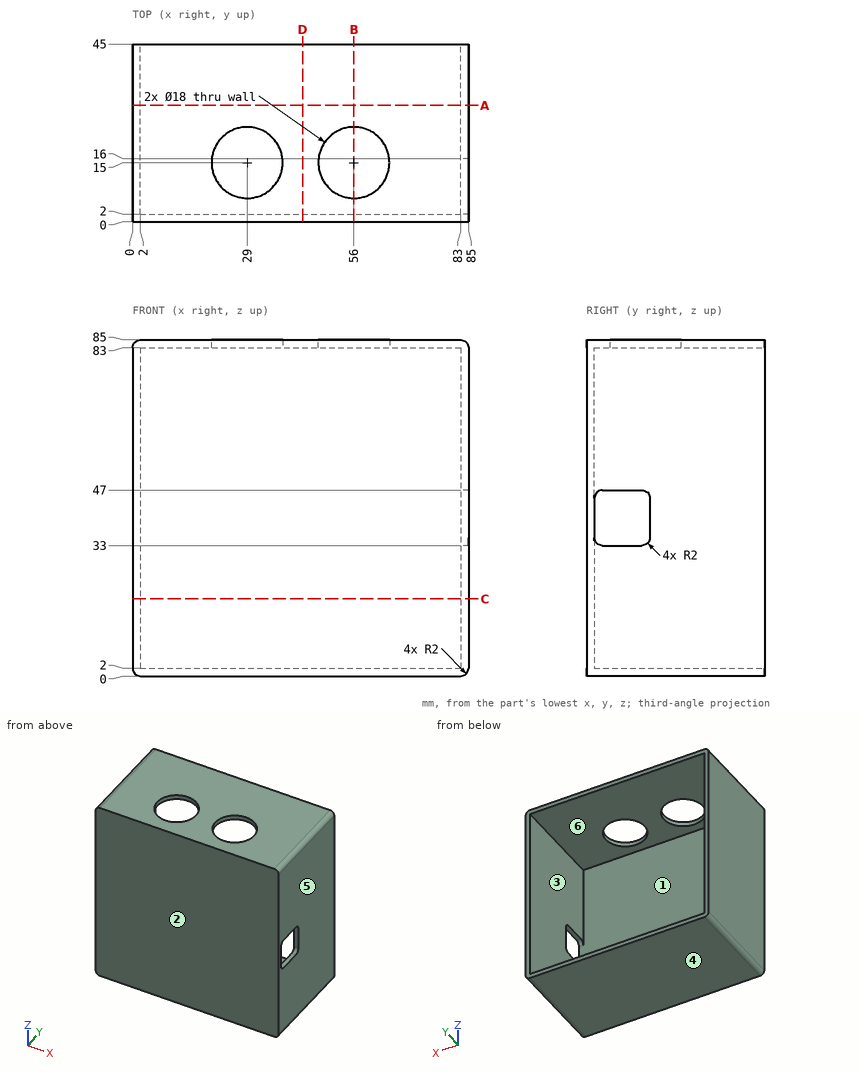
Answer from the drawing. Dimensions are ordinates in mm from the lowest x, y and z of the part. A direction names the side the tool comes from. Give positions to 0.01 mm unless a question says otherwise; leave off trailing zeros. Loops run counter-clockwise (first coordinate to the right, second up) from the corner with the lowest first, then second, coordinate; pieces in that order, holes last. Notation, with made-up numbers: (-19, 39) -> (-11, 39) arc R23 ccw to (-11, 48) -> close; hole circle Ø7 at (72.25, -27). An arc over 180 degrees is marked (long way). One line per question, with ' | ' between items. Start each with the question number.
1) Section C-C, the plane z = 19.5 is taken. Determine the outline of the cut face in (x, y), then the cut area to 3 significant figures.
2) For the marked faces 5 and 6, determine the directions among +Z, -Z, +X, -X, +Y, -Y from which every point of the face is accessible in a straight line to the end or side of a thin tool.
3) Section A-A, the plane y = 29.5 is taken. Determine the outline of the cut face in (x, z).
4) Determine the mould class of the marked faces 1, 2, 3 and 4 for opening direction Z: +Z half, -Z half, draft (parallel to the pull), parting line (faces both ways), or undercut.
5) Section D-D, the plane x = 43 is taken. Determine the outline of the cut face in (y, z), then the cut area to 3 significant figures.
6) Each of these flat-tipped pins is pushed along its axis until it touches: pin 1 (0.6 mm diameter, centred on x = 84.5, y = 8, fed in from +Z); pin 2 (1 mm diameter, centred on x = 84.5, y = 9.5, fed in from -Z); pin 3 (2 mm diameter, centred on x = 60, z = 54, fed in from +Y). Where does it stop, or does it pass through?
7) Section B-B, the plane x = 56 is taken. Determine the outline of the cut face in (y, z), then the cut area to 3 significant figures.
8) Straight lines are drawn through the part: L1, parallel to Y at x = 29, z = 83.9; L2, parallel to Z at x = 73, y = 29. For each, find the intervals that lie inside material, in ascending order.
Resolved:
1) outline: (0, 0) -> (85, 0) -> (85, 45) -> (83, 45) -> (83, 2) -> (2, 2) -> (2, 45) -> (0, 45) -> close | area: 342 mm2
2) face 5: +Z, -Z, +X, +Y, -Y | face 6: +Y
3) outline: (0, 2) arc R2 ccw to (2, 0) -> (83, 0) arc R2 ccw to (85, 2) -> (85, 83) arc R2 ccw to (83, 85) -> (2, 85) arc R2 ccw to (0, 83) -> close; hole (2, 2) -> (83, 2) -> (83, 83) -> (2, 83) -> close
4) face 1: undercut | face 2: draft | face 3: undercut | face 4: -Z half
5) outline: (0, 0) -> (45, 0) -> (45, 2) -> (2, 2) -> (2, 83) -> (45, 83) -> (45, 85) -> (0, 85) -> close | area: 342 mm2
6) pin 1: z = 84.6 | pin 2: z = 0.27 | pin 3: y = 2
7) outline: (0, 0) -> (45, 0) -> (45, 2) -> (2, 2) -> (2, 83) -> (6, 83) -> (6, 85) -> (0, 85) -> close; (24, 83) -> (45, 83) -> (45, 85) -> (24, 85) -> close | area: 306 mm2
8) L1: 0 to 6, 24 to 45 | L2: 0 to 2, 83 to 85
